from build123d import *

# Parameters (mm, degrees)
MODEL_R             = 1.230314961
MODEL_R_2           = 0.492125984
MODEL_R_3           = 0.246062992
BOSS_EXTRUDE1_DEPTH = 3


with BuildPart() as part:
    # Model → Boss-Extrude1 (new body)
    with BuildSketch(Plane.XY):
        Polygon((0, 0), (10, 0), (10, 12.5), (9.99048659, 12.71788878), (9.962020177, 12.93411971), (9.914816068, 13.147047244), (9.849231053, 13.355050443), (9.765769562, 13.556545276), (9.665062131, 13.75), (9.547880782, 13.933941314), (9.415111344, 14.106969734), (9.267765748, 14.267765748), (9.106969734, 14.415111344), (8.933941314, 14.547880782), (8.75, 14.665062131), (8.556545276, 14.765769562), (8.355050443, 14.849231053), (8.147047244, 14.914816068), (7.93411971, 14.962020177), (7.71788878, 14.99048659), (7.5, 15), (2.5, 15), (2.28211122, 14.99048659), (2.06588029, 14.962020177), (1.852952756, 14.914816068), (1.644949557, 14.849231053), (1.443454724, 14.765769562), (1.25, 14.665062131), (1.066058686, 14.547880782), (0.893030266, 14.415111344), (0.732234252, 14.267765748), (0.584888656, 14.106969734), (0.452119218, 13.933941314), (0.334937869, 13.75), (0.234230438, 13.556545276), (0.150768947, 13.355050443), (0.085183932, 13.147047244), (0.037979823, 12.93411971), (0.00951341, 12.71788878), (0, 12.5), align=None)
        with Locations((5, 12.5)):
            Circle(MODEL_R, mode=Mode.SUBTRACT)
        with Locations((8.75, 2.5)):
            Circle(MODEL_R_2, mode=Mode.SUBTRACT)
        with Locations((6.25, 2.5)):
            Circle(MODEL_R_2, mode=Mode.SUBTRACT)
        with Locations((3.75, 2.5)):
            Circle(MODEL_R_2, mode=Mode.SUBTRACT)
        with Locations((1.25, 2.5)):
            Circle(MODEL_R_2, mode=Mode.SUBTRACT)
        with Locations((1.125, 9.25)):
            Circle(MODEL_R_3, mode=Mode.SUBTRACT)
        with Locations((8.5, 10.875)):
            Circle(MODEL_R_3, mode=Mode.SUBTRACT)
        with Locations((7, 10.875)):
            Circle(MODEL_R_3, mode=Mode.SUBTRACT)
    extrude(amount=BOSS_EXTRUDE1_DEPTH)


solid = part.part
Design review of the part built by this model. Coordinates are the model's own, in mm. Coordinates: 2 decimals unless noted, no trailing zeros. Order: outer loops, then holes, each group sorted by start corner. A loop starts at its lowest first (then second) coordinate and runs counter-clockwise, first axis right, second up. Notation, with made-up numbers: (49.5, 83) -> (102.5, 83) arc R24 ccw to (102.5, 103) -> close; hole circle Ø10 at (27.5, 20). An arc over 180 degrees is marked (long way). Use one line per item in the form item = value. Start each with the question number.
(1) For probe 1 along Y at (x, z) = (7, 2.45); probe 2 along Y at (x, z) = (1.25, 1.15); probe 3 along Y at (x, z) = (1, 0.7), list the stretches that pass through material, from the lowest coordinate up.
(2) The part is to be moulded in two halves that separate along Y. For faces 1 (the cylindrical face through (4.024, 11.751, 1.479)), 2 (the flat face through (5, 0, 1)), 3 (the flat face through (5, 15, 1)), 4 (the flat face through (5, 8, 0)), say which applies: +Y half, -Y half, draft (parallel to the pull), parting line (faces both ways), or undercut.
(3) Add section A-A on y = 2.5. State the section outline as (x, z) points.
(4) Add section D-D on x = 6. State the section outline as (y, z) points, plus the area to 3 significant figures.
(5) Add section B-B on x = 7. State the section outline as (y, z) points, plus the area to 3 significant figures.
(6) Add section C-C on y = 9.25. State the section outline as (x, z) points.
Answer block:
q1.probe_1 = 0 to 10.63, 11.12 to 15
q1.probe_2 = 0 to 2.01, 2.99 to 9.04, 9.46 to 14.67
q1.probe_3 = 0 to 2.08, 2.92 to 9.04, 9.46 to 14.5
q2.face_1 = undercut
q2.face_2 = -Y half
q2.face_3 = +Y half
q2.face_4 = draft
q3.outline = (0, 0) -> (0.76, 0) -> (0.76, 3) -> (0, 3) -> close; (1.74, 0) -> (3.26, 0) -> (3.26, 3) -> (1.74, 3) -> close; (4.24, 0) -> (5.76, 0) -> (5.76, 3) -> (4.24, 3) -> close; (6.74, 0) -> (8.26, 0) -> (8.26, 3) -> (6.74, 3) -> close; (9.24, 0) -> (10, 0) -> (10, 3) -> (9.24, 3) -> close
q4.outline = (0, 0) -> (2.08, 0) -> (2.08, 3) -> (0, 3) -> close; (2.92, 0) -> (11.78, 0) -> (11.78, 3) -> (2.92, 3) -> close; (13.22, 0) -> (15, 0) -> (15, 3) -> (13.22, 3) -> close
q4.area = 38.2 mm²
q5.outline = (0, 0) -> (10.63, 0) -> (10.63, 3) -> (0, 3) -> close; (11.12, 0) -> (15, 0) -> (15, 3) -> (11.12, 3) -> close
q5.area = 43.5 mm²
q6.outline = (0, 0) -> (0.88, 0) -> (0.88, 3) -> (0, 3) -> close; (1.37, 0) -> (10, 0) -> (10, 3) -> (1.37, 3) -> close
